For this review, take the finished solid that the model builds, in its own axes (mm). A direction names the side the tool comes from. Coordinates: 2 decimals unless noted, no trailing zeros. Write each loop counter-clockwise with the first axis right and the second up, starting at its lowest first coordinate (ties: lowest second). Pieces come first, ordered by that corner, then holes.
```python
from build123d import *

# Parameters (mm, degrees)
F6_W     = 63.5
F6_H     = 6.35
F0_DEPTH = 123.825
F3_W     = 152.4
F3_H     = 101.6
F4_DEPTH = 6.35
F5_R     = 5.08


with BuildPart() as f0:
    # F6 (on Front) → F0 (new body)
    with BuildSketch(Plane.XZ):
        with Locations((38.1, 22.225)):
            Rectangle(F6_W, F6_H)
    extrude(amount=F0_DEPTH)

    # F1: F0 across plane


with BuildPart() as f0_1:
    add(f0.part)
    add(f0.part.mirror(Plane.XZ))

    # F2: F0 across plane


with BuildPart() as f0_2:
    add(f0_1.part)
    add(f0_1.part.mirror(Plane.XZ))

    # F3 (on Right) → F4 (join)
    with BuildSketch(Plane.YZ):
        with Locations((0, -25.4)):
            Rectangle(F3_W, F3_H)
        with BuildLine():
            ThreePointArc((-50.8, -63.5), (-55.2901280605, -61.6401280605), (-57.15, -57.15))
            Line((-57.15, -57.15), (-57.15, -25.4))
            ThreePointArc((-57.15, -25.4), (-50.8, -19.05), (-44.45, -25.4))
            Line((-44.45, -25.4), (-44.45, -57.15))
            ThreePointArc((-44.45, -57.15), (-46.3098719395, -61.6401280605), (-50.8, -63.5))
        make_face(mode=Mode.SUBTRACT)
        with BuildLine():
            ThreePointArc((50.8, -63.5), (46.3098719395, -61.6401280605), (44.45, -57.15))
            Line((44.45, -57.15), (44.45, -25.4))
            ThreePointArc((44.45, -25.4), (50.8, -19.05), (57.15, -25.4))
            Line((57.15, -25.4), (57.15, -57.15))
            ThreePointArc((57.15, -57.15), (55.2901280605, -61.6401280605), (50.8, -63.5))
        make_face(mode=Mode.SUBTRACT)
    extrude(amount=F4_DEPTH)

    # F5
    f5_edges = [f0_2.edges().sort_by_distance(p)[0] for p in [
        (0, 0, 25.4),
        (38.1, 123.825, 25.4),
        (38.1, -123.825, 25.4),
    ]]
    fillet(f5_edges, radius=F5_R)


solid = f0_2.part
```
1) Consider section C-C (x = 32). Give the boundary of the cut face in (y, z) (3 decimals), then the cut area to 3 significant figures.
2) Consider section B-B (y = -26.5). Give the boundary of the cut face in (x, z).
3) For L1, parallel to Z at x = 10.5, y = -99; L2, parallel to X at y = 36.5, z = -6, list the stretches that pass through material, from the lowest coordinate up.
4) Consider section A-A (z = -48.5). Give the boundary of the cut face in (x, y).
5) Clearance check with flat-ended pins moving along their axes: P1, Ø3, axis at x = 4, z = -48, coming from the -Y side; P2, Ø1.9, axis at x = 3, z = -40, coming from the +Y side; P3, Ø5, axis at y = -91, z = 21.5, coming from the -X side. State where each tip first meets the part, or that it passes through.
6) Consider section D-D (z = -23). Give the boundary of the cut face in (x, y), then the cut area to 3 significant figures.
7) The part is to be moulded in two halves that separate along Z. For faces 5 (the face through (38, -2, 19.05)), 6 (the face through (3.13, 50.66, -19.05)), 7 (the face through (1.528, 1.067, 23.951)), say which applies: pulls with the +Z half, pulls with the -Z half, needs draft (parallel to the pull), parting line crosses it, or undercut.
8) Tool access review of faces 1 (the face through (3, -57.15, -41)), 2 (the face through (6.35, 100, 22)), 3 (the face through (6.35, -1, -28)), 4 (the face through (6.35, -100, 22)): name each direction out of +Z, -Z, +X, -X, +Y, -Y from which nothing blocks a thin tool from reaching the whole face with its end or side.
Results:
1. outline: (-123.825, 19.05) - (123.825, 19.05) - (123.825, 20.32) arc R5.08 ccw to (118.745, 25.4) - (-118.745, 25.4) arc R5.08 ccw to (-123.825, 20.32) - close
1. area: 1,560 mm2
2. outline: (0, -76.2) - (6.35, -76.2) - (6.35, 19.05) - (69.85, 19.05) - (69.85, 25.4) - (5.08, 25.4) arc R5.08 ccw to (0, 20.32) - close
3. L1: z = 19.05 to 25.4
3. L2: x = 0 to 6.35
4. outline: (0, -76.2) - (6.35, -76.2) - (6.35, -57.15) - (0, -57.15) - close; (0, -44.45) - (6.35, -44.45) - (6.35, 44.45) - (0, 44.45) - close; (0, 57.15) - (6.35, 57.15) - (6.35, 76.2) - (0, 76.2) - close
5. P1: stops at y = -76.2
5. P2: stops at y = 76.2
5. P3: stops at x = 6.35
6. outline: (0, -76.2) - (6.35, -76.2) - (6.35, -56.68) - (0, -56.68) - close; (0, -44.92) - (6.35, -44.92) - (6.35, 44.92) - (0, 44.92) - close; (0, 56.68) - (6.35, 56.68) - (6.35, 76.2) - (0, 76.2) - close
6. area: 818 mm2
7. face 5: pulls with the -Z half
7. face 6: undercut
7. face 7: pulls with the +Z half
8. face 1: +X, -X
8. face 2: +Z, -Z, -X, +Y
8. face 3: -Z, +X, +Y, -Y
8. face 4: +Z, -Z, -X, -Y
